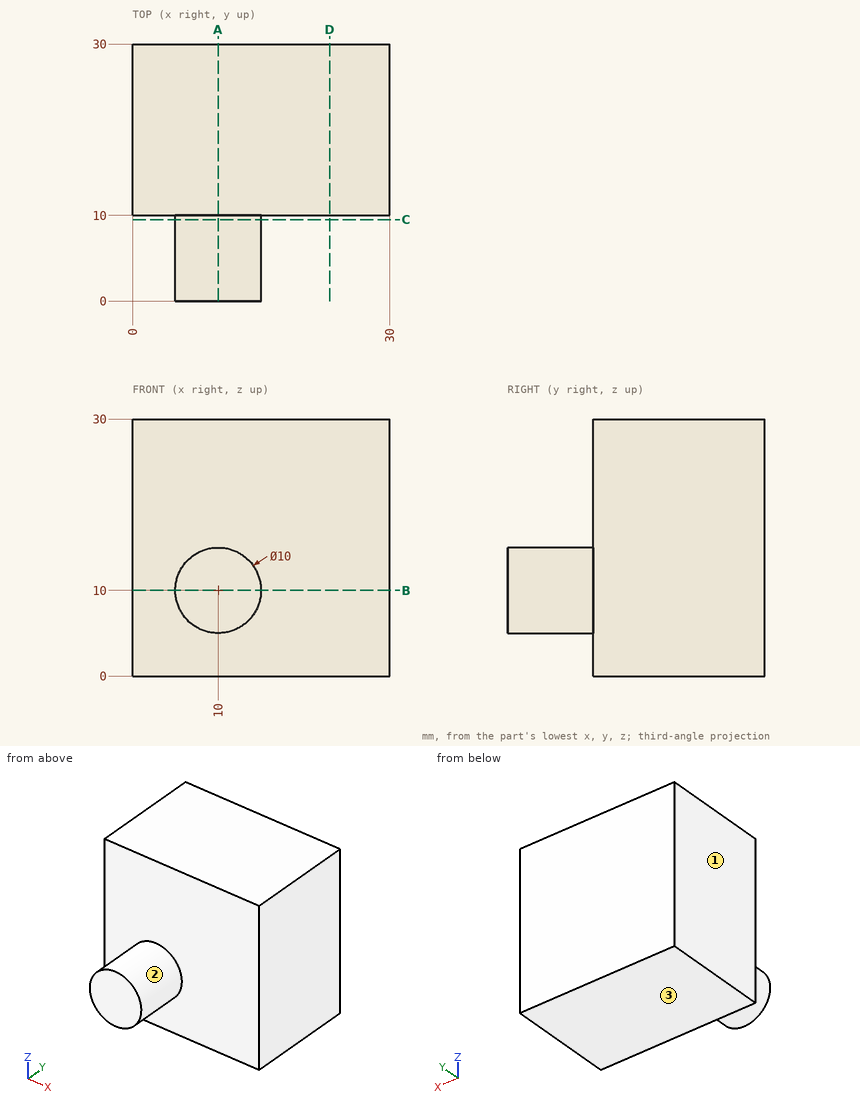
Here's the drawing with two shaded views (mm, measured from the low corner). I have some questions. Give positions to 0.01 mm unless a question says otherwise; leave off trailing zeros. Order: outer loops, then holes, each group sorted by start corner. A loop starts at its lowest first (then second) coordinate and runs counter-clockwise, first axis right, second up.
Q1. If I drill on line 1 along Y through (x, z) = (15.5, 10.5); line 2 along X through (y, z) = (4.5, 13.75), over which ranges is the centre line in solid material (lowest first)?
Q2. Suppose I cut it at A-A, the plane x = 10. Write out the boundary of the cut face in (y, z).
Q3. Suppose I cut it at D-D, the plane x = 23. Write out the boundary of the cut face in (y, z), and give its area (3 significant figures).
Q4. Suppose I cut it at C-C, the plane y = 9.5. Write out the boundary of the cut face in (x, z), and give its area (3 significant figures).
Q5. Suppose I cut it at B-B, the plane z = 10. Write out the boundary of the cut face in (x, y).
Q6. We'd pull the mould along Z, two halves only. Please class the marked faces 1, 2 and 3: +Z half, -Z half, draft (parallel to the pull), parting line (faces both ways), or undercut.
Q7. I'm going to push a flat-ended pin straight in: P1, Ø9, axis at x = 12, z = 18, coming from the -Y side. Where does the tip first touch, or does it pass through?
Solution:
1. line 1: y = 10 to 30
1. line 2: x = 6.69 to 13.31
2. outline: (0, 5) - (10, 5) - (10, 0) - (30, 0) - (30, 30) - (10, 30) - (10, 15) - (0, 15) - close
3. outline: (10, 0) - (30, 0) - (30, 30) - (10, 30) - close
3. area: 600 mm2
4. outline: circle Ø10 at (10, 10)
4. area: 78.5 mm2
5. outline: (0, 10) - (5, 10) - (5, 0) - (15, 0) - (15, 10) - (30, 10) - (30, 30) - (0, 30) - close
6. face 1: draft
6. face 2: parting line
6. face 3: -Z half
7. P1: stops at y = 0
